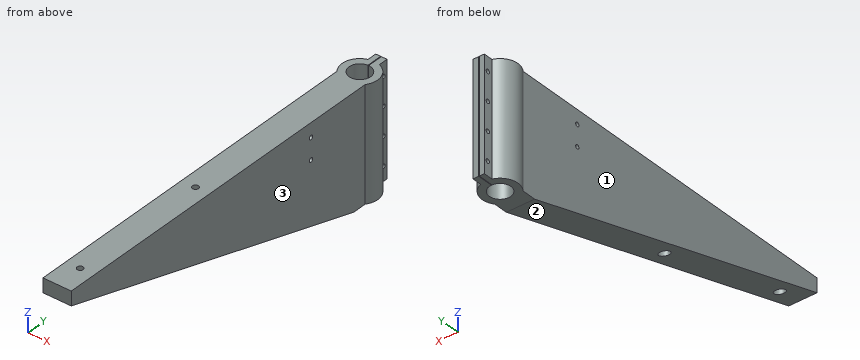
from build123d import *

# Parameters (mm, degrees)
F1_DEPTH  = 80
F0_R      = 7.6
F2_DEPTH  = 80
F3_R      = 2.15
F4_DEPTH  = 80.001
F5_R      = 3.65
F5_R_2    = 2.15
F6_DEPTH  = 70
F8_DEPTH  = 22.601
F10_DEPTH = 80.001
F11_R     = 1.45
F12_DEPTH = 16.601
F13_R     = 1.45
F14_DEPTH = 22.601


with BuildPart() as f1:
    # F0 (on Top) → F1 (new body)
    with BuildSketch(Plane.XY):
        with BuildLine():
            ThreePointArc((10, -7.6655071587), (0, -12.6), (-10, -7.6655071587))
            Line((-10, -7.6655071587), (-10, -262.6))
            Line((-10, -262.6), (10, -262.6))
            Line((10, -262.6), (10, -7.6655071587))
        make_face()
    extrude(amount=-F1_DEPTH)

    # F0 (on Top) → F2 (join)
    with BuildSketch(Plane.XY):
        with BuildLine():
            Line((-4, 18.6), (-4, 11.948221625))
            ThreePointArc((-4, 11.948221625), (-12.0488418199, 3.685839226), (-10, -7.6655071587))
            ThreePointArc((-10, -7.6655071587), (0, -12.6), (10, -7.6655071587))
            ThreePointArc((10, -7.6655071587), (12.0488418199, 3.685839226), (4, 11.948221625))
            Line((4, 11.948221625), (4, 18.6))
            Line((4, 18.6), (-4, 18.6))
        make_face()
        Circle(F0_R, mode=Mode.SUBTRACT)
    extrude(amount=-F2_DEPTH)

    # F3 (on face) → F4 (cut, through all)
    with BuildSketch(Plane.XY):
        with Locations((0, -142.6)):
            Circle(F3_R)
        with Locations((0, -242.6)):
            Circle(F3_R)
    extrude(amount=-F4_DEPTH, mode=Mode.SUBTRACT)

    # F5 (on face) → F6 (cut)
    with BuildSketch(Plane(origin=(0, 0, -80), x_dir=(1, 0, 0), z_dir=(0, 0, -1))):
        with Locations((0, 242.6)):
            Circle(F5_R)
        with Locations((0, 242.6)):
            Circle(F5_R_2, mode=Mode.SUBTRACT)
        with Locations((0, 142.6)):
            Circle(F5_R)
        with Locations((0, 142.6)):
            Circle(F5_R_2, mode=Mode.SUBTRACT)
    extrude(amount=-F6_DEPTH, mode=Mode.SUBTRACT)

    # F7 (on face) → F8 (cut, through all)
    with BuildSketch(Plane.YZ.offset(10)):
        Polygon((-262.6, -80), (-17.6655071587, -80), (-262.6, -10), align=None)
    extrude(amount=-F8_DEPTH, mode=Mode.SUBTRACT)

    # F9 (on face) → F10 (cut, through all)
    with BuildSketch(Plane.XY):
        with BuildLine():
            Line((0, 7.6), (0, 18.6))
            Line((0, 18.6), (-0.5, 18.6))
            Line((-0.5, 18.6), (-0.5, 7.5835347959))
            ThreePointArc((-0.5, 7.5835347959), (-0.2501355147, 7.5958825836), (0, 7.6))
        make_face()
        with BuildLine():
            ThreePointArc((0.5, 7.5835347959), (0.2501355147, 7.5958825836), (0, 7.6))
            Line((0, 7.6), (0, 0))
            Line((0, 0), (0.5, 0))
            Line((0.5, 0), (0.5, 7.5835347959))
        make_face()
        with BuildLine():
            Line((0, 0), (0, 7.6))
            ThreePointArc((0, 7.6), (-0.2501355147, 7.5958825836), (-0.5, 7.5835347959))
            Line((-0.5, 7.5835347959), (-0.5, 0))
            Line((-0.5, 0), (0, 0))
        make_face()
    extrude(amount=-F10_DEPTH, mode=Mode.SUBTRACT)

    # F11 (on face) → F12 (cut, through all)
    with BuildSketch(Plane.YZ.offset(4)):
        with Locations((15.6, -30)):
            Circle(F11_R)
        with Locations((15.6, -70)):
            Circle(F11_R)
        with Locations((15.6, -50)):
            Circle(F11_R)
        with Locations((15.6, -10)):
            Circle(F11_R)
    extrude(amount=-F12_DEPTH, mode=Mode.SUBTRACT)

    # F13 (on face) → F14 (cut, through all)
    with BuildSketch(Plane.YZ.offset(10)):
        with Locations((-54.6655071587, -10)):
            Circle(F13_R)
        with Locations((-54.6655071587, -25)):
            Circle(F13_R)
    extrude(amount=-F14_DEPTH, mode=Mode.SUBTRACT)


solid = f1.part
Work out the finished part from the listing and answer in its coordinate system (mm). Face numbers are marked on the shaded views. A direction names the side the tool comes from. Round coordinates to 2 decimals unless told otherwise and drop trailing zeros. Write each loop counter-clockwise with the first axis right and the second up, starting at its lowest first coordinate (ties: lowest second). Pieces come first, ordered by that corner, then holes.
1) Given pin 1 Ø1 at (x, y) = (4.5, -145) entering from -Z; pin 2 Ø3.5 at (y, z) = (15.6, -70) entering from -X; pin 3 Ø13.5 at (x, y) = (0, 0) entering from +Z; pin 4 Ø12 at (y, z) = (15.5, -29) entering from +X, each flat-ended and moving along its own axis, determine where each tip first touches the part or whether it passes through.
2) A cutting plane is placed at D-D (y = -35.5). Give the vertices of the cut face in (x, z).
3) A cutting plane is placed at B-B (z = -62). Give the vertices of the cut face in (x, y), plus the area to 3 significant figures.
4) Straight lines are drawn through the part: line 1 (X direction, y = -142, z = -35); line 2 (Z direction, x = -9.5, y = -55); line 3 (Z direction, x = 0.25, y = -54). For each, find the intervals that lie inside material, in ascending order.
5) A tool of negligible diameter and unlimited length cuts with its end or side. For the marked faces 1, 2 and 3, from which of +Z, -Z, +X, -X, +Y, -Y can it reach the whole face along a straight path? Write none if from no direction.
6) A cutting plane is placed at C-C (y = -165.5). Give the vertices of the cut face in (x, z), plus the area to 3 significant figures.
7) A cutting plane is placed at A-A (y = 0). Give the vertices of the cut face in (x, z), plus the area to 3 significant figures.
Completed:
1. pin 1: stops at z = -43.75
1. pin 2: stops at x = -4
1. pin 3: passes through
1. pin 4: stops at x = 8.28
2. outline: (-10, -74.9) - (10, -74.9) - (10, 0) - (-10, 0) - close
3. outline: (-10, -80.65) - (10, -80.65) - (10, -7.67) arc R12.6 ccw to (4, 11.95) - (4, 18.6) - (0, 18.6) - (0, 7.6) arc R7.6 cw (long way) to (-0.5, 7.58) - (-0.5, 18.6) - (-4, 18.6) - (-4, 11.95) arc R12.6 ccw to (-10, -7.67) - close
3. area: 1,750 mm2
4. line 1: x = -10 to -3.6, 3.6 to 10
4. line 2: z = -69.33 to -26.41, -23.59 to -11.41, -8.59 to 0
4. line 3: z = -69.62 to -26.29, -23.71 to -11.29, -8.71 to 0
5. face 1: +Z, -Z, -X, -Y
5. face 2: -Z, +X, -X, -Y
5. face 3: +Z, -Z, +X, -Y
6. outline: (-10, -37.75) - (10, -37.75) - (10, 0) - (-10, 0) - close
6. area: 755 mm2
7. outline: (-12.6, -80) - (-7.6, -80) - (-7.6, 0) - (-12.6, 0) - close; (7.6, -80) - (12.6, -80) - (12.6, 0) - (7.6, 0) - close
7. area: 800 mm2
